```python
from build123d import *

# Parameters (mm, degrees)
TAP_DRILL_FOR_3_8_16_TAP1_D = 10.0838
CIRPATTERN1_COUNT           = 10


with BuildPart() as part:
    # Sketch1 → Revolve1 (revolve)
    with BuildSketch(Plane.XY, mode=Mode.PRIVATE) as revolve1_sk:
        Polygon((51.1302, 0), (51.1302, -220.345), (53.6702, -220.345), (53.6702, -223.393), (51.1302, -223.393), (51.1302, -234.95), (57.15, -234.95), (57.15, -6.35), (76.2, -6.35), (76.2, 0), align=None)
    revolve(revolve1_sk.sketch.rotate(Axis((0, 0, 0), (0, -1, 0)), 180), axis=Axis((0, 0, 0), (0, -1, 0)))

    # Tap Drill for 3/8-16 Tap1 (through all)
    with Locations(Plane(origin=(0, 0, 0), x_dir=(1, 0, 0), z_dir=(0, 1, 0))):
        with Locations((67.31, 0)):
            tap_drill_for_3_8_16_tap1 = Hole(TAP_DRILL_FOR_3_8_16_TAP1_D / 2)

    # CirPattern1: Tap Drill for 3/8-16 Tap1 ×10 about axis
    cirpattern1_axis = Axis((0, 0, 0), (0, 1, 0))
    for i in range(1, CIRPATTERN1_COUNT):
        add(tap_drill_for_3_8_16_tap1.rotate(cirpattern1_axis, i * 360 / CIRPATTERN1_COUNT), mode=Mode.SUBTRACT)


solid = part.part
```
Geometry: final body of the model. Coordinates: model frame, mm. A direction names the side the tool comes from. Coordinates: 2 decimals unless noted, no trailing zeros. Write each loop counter-clockwise with the first axis right and the second up, starting at its lowest first coordinate (ties: lowest second). Pieces come first, ordered by that corner, then holes. Notation, with made-up numbers: M -18.5,-30 L 33.5,-30 A11 ccw 33.5,-15 Z; hole C 81,29.5 d3. An arc over 180 degrees is marked long. Use CSV: the item, a comma, the result in double quotes. Start each with the question number.
1. Cut plane A-A on z = 0. Return the cut outline in (x, y) (3 decimals), plus the area to 3 significant figures.
2. Cut plane D-D on z = -62. Return the cut outline in (x, y), plus the area to 3 significant figures.
3. Reachability of faces 1 (the face through (11, -6.35, -57)), 2 (the face through (47.5, -220.345, 19.6)), 3 (the face through (71.31, -3.22, 3.07)) from +Z, -Z, +X, -X, +Y, -Y: full face, straight path, thin tool, end or side. Return the list, or none.
4. Cut plane B-B on x = 46.5. Return the cut outline in (y, z) (3 decimals), plus the area to 3 significant figures.
5. Ray query, probe 1 along Z at (x, y) = (0, -221.8); probe 2 along Y at (x, z) = (-20.5, -48.5) (3 decimals); probe 3 along Z at (x, y) = (-32, -43). Return the intervals inside material, ascending.
6. First-contact query: P1, Ø8, axis at x = 23.5, y = -163, coming from the +Z side; P2, Ø2, axis at y = -62, z = 17, coming from the +X side; P3, Ø1, axis at y = -185, z = -58.5, coming from the +X side; P4, Ø10, axis at y = -71.5, z = -11.5, coming from the +X side. Flat tips, straight axial feed; report the tip coordinate or a pass-through.
7. Cut plane C-C on z = -31.5. Return the cut outline in (x, y) (3 decimals), plus the area to 3 significant figures.
8. Mould query, pull axis Z, two halves, no side actions, for faces 4 (the face through (-43, -234.95, 29)), 5 (the face through (57.095, -119.05, -2.513)), 6 (the face through (-49.763, -3.219, 41.41)). Classes: pulls with the +Z half, pulls with the -Z half, needs draft (parallel to the pull), parting line crosses it, or undercut.
Entries:
1,outline,"M -76.2,-6.35 L -72.352,-6.35 L -72.352,0 L -76.2,0 Z; M -62.268,-6.35 L -57.15,-6.35 L -57.15,-234.95 L -51.13,-234.95 L -51.13,-223.393 L -53.67,-223.393 L -53.67,-220.345 L -51.13,-220.345 L -51.13,0 L -62.268,0 Z; M 51.13,-234.95 L 57.15,-234.95 L 57.15,-6.35 L 62.268,-6.35 L 62.268,0 L 51.13,0 L 51.13,-220.345 L 53.67,-220.345 L 53.67,-223.393 L 51.13,-223.393 Z; M 72.352,-6.35 L 76.2,-6.35 L 76.2,0 L 72.352,0 Z"
1,area,"2,930 mm²"
2,outline,"M -44.3,-6.35 L -25.42,-6.35 L -25.42,0 L -44.3,0 Z; M -16.18,-6.35 L 16.18,-6.35 L 16.18,0 L -16.18,0 Z; M 25.42,-6.35 L 44.3,-6.35 L 44.3,0 L 25.42,0 Z"
2,area,"445 mm²"
3,face 1,"-Y"
3,face 2,"none"
3,face 3,"+Y, -Y"
4,outline,"M -234.95,-33.225 L -6.35,-33.225 L -6.35,-60.367 L 0,-60.367 L 0,-21.261 L -220.345,-21.261 L -220.345,-26.8 L -223.393,-26.8 L -223.393,-21.261 L -234.95,-21.261 Z; M -234.95,21.261 L -223.393,21.261 L -223.393,26.8 L -220.345,26.8 L -220.345,21.261 L 0,21.261 L 0,60.367 L -6.35,60.367 L -6.35,33.225 L -234.95,33.225 Z"
4,area,"5,930 mm²"
5,probe 1,"-57.15 to -53.67, 53.67 to 57.15"
5,probe 2,"-234.95 to -223.393, -220.345 to 0"
5,probe 3,"-47.35 to -39.88, 39.88 to 47.35"
6,P1,"z = 53.72"
6,P2,"x = 54.86"
6,P3,"through"
6,P4,"x = 56.78"
7,outline,"M -69.384,-6.35 L -47.685,-6.35 L -47.685,-234.95 L -40.275,-234.95 L -40.275,-223.393 L -43.454,-223.393 L -43.454,-220.345 L -40.275,-220.345 L -40.275,0 L -69.384,0 Z; M 40.275,-234.95 L 47.685,-234.95 L 47.685,-6.35 L 69.384,-6.35 L 69.384,0 L 40.275,0 L 40.275,-220.345 L 43.454,-220.345 L 43.454,-223.393 L 40.275,-223.393 Z"
7,area,"3,740 mm²"
8,face 4,"needs draft"
8,face 5,"parting line crosses it"
8,face 6,"undercut"
